Design review of the part built by this model. Coordinates are the model's own, in mm. A direction names the side the tool comes from. Coordinates: 2 decimals unless noted, no trailing zeros. Loops run counter-clockwise (first coordinate to the right, second up) from the corner with the lowest first, then second, coordinate; pieces in that order, holes last. Notation, with made-up numbers: (69, -38) - (75, -38) arc R28 cw to (75, -4) - close; hole circle Ø10 at (81, 45). An arc over 180 degrees is marked (long way). Return JSON: item names as keys, results as strings. Group by question number.
from build123d import *

# Parameters (mm, degrees)
FILLET1_R = 10


with BuildPart() as part:
    # Sketch1 → Revolve1 (revolve)
    with BuildSketch(Plane.XY):
        with BuildLine():
            ThreePointArc((1.5, 24.57), (4.516916983, 31.065059709), (11.426070736, 32.949518021))
            ThreePointArc((11.426070736, 32.949518021), (54.755418646, 28.809847984), (98.05771623, 33.223495257))
            Line((98.05771623, 33.223495257), (124.713836064, 28.549572437))
            Line((124.713836064, 28.549572437), (162.227403624, 13.5))
            Line((162.227403624, 13.5), (174.917066057, 13.5))
            Line((174.917066057, 13.5), (176.417066057, 13.5))
            Line((176.417066057, 13.5), (176.417066057, 15))
            Line((176.417066057, 15), (162.517066057, 15))
            Line((162.517066057, 15), (125.127066057, 30))
            Line((125.127066057, 30), (98.037066057, 34.75))
            ThreePointArc((98.037066057, 34.75), (54.883168803, 30.3102994), (11.697066057, 34.424946311))
            ThreePointArc((11.697066057, 34.424946311), (3.556812147, 32.217570221), (0, 24.57))
            Line((0, 24.57), (0, 0))
            Line((0, 0), (1.5, 0))
            Line((1.5, 0), (1.5, 24.57))
        make_face()
    revolve(axis=Axis((174.917066057, 0, 0), (-1, 0, 0)))

    # Fillet1
    fillet1_edges = [part.edges().sort_by_distance(p)[0] for p in [
        (98.037066057, -34.75, 0),
        (125.127066057, -30, 0),
        (162.517066057, -15, 0),
    ]]
    fillet(fillet1_edges, radius=FILLET1_R)


solid = part.part
Item 1: For faces 1 (the face through (176.417, 11.18, -7.85)), 2 (the face through (117.496, 28.438, -8.956)), 3 (the face through (169.42, -2.93, 13.18)), list the 3-axis set-ups (+Z, -Z, +X, -X, +Y, -Y) from which the entire face can be reached by the end or side of a thin tool; tool diameter is ignored.
Item 2: Add section A-A (x = 118). State the section outline as (y, z) points.
Item 3: Draft analysis for pull direction Y (two halves, no side actions). For faces 4 (the face through (170.349, 13.856, 5.745)), 5 (the face through (0, 0, 0)), 6 (the face through (152.07, -13.95, 10.69)), state which applies: pulls with the +Y half, pulls with the -Y half, needs draft (parallel to the pull), parting line crosses it, or undercut.
Item 4: Add section B-B (x = 157.5). State the section outline as (y, z) points.
Item 5: For P1, Ø2, axis at x = 78.5, z = 6, coming from the +Y side; P2, Ø12, axis at x = 109, z = -15.5, coming from the +Y side; P3, Ø1, axis at x = 69.5, z = -12.5, coming from the +Y side, all flat-tipped, find the tip position at first contact; note any pin that passes through.
Item 6: To check wall thickness, follow line 1 (Y direction, x = 166.5, z = 0); line 2 (Y direction, x = 18, z = 11.5). State the ranges of each line that lie inside material, in increasing order. Write a range as from..to.
Answers below:
{
 "1": {"face 1": "+Z, -Z, +X, +Y, -Y", "face 2": "none", "face 3": "+X"},
 "2": {"outline": "circle Ø62.5 at (0, 0); hole circle Ø59.45 at (0, 0)"},
 "3": {"face 4": "parting line crosses it", "face 5": "needs draft", "face 6": "undercut"},
 "4": {"outline": "circle Ø34.03 at (0, 0); hole circle Ø30.79 at (0, 0)"},
 "5": {"P1": "stops at y = 31.31", "P2": "stops at y = 31.72", "P3": "stops at y = 28.43"},
 "6": {"line 1": "y = -15..-13.5, 13.5..15", "line 2": "y = -31.23..-29.61, 29.61..31.23"}
}
